```python
from build123d import *

# Parameters (mm, degrees)
F1_DEPTH = 9


with BuildPart() as f1:
    # F0 (on Front) → F1 (new body)
    with BuildSketch(Plane.XZ):
        with BuildLine():
            ThreePointArc((-19.7199515168, 22.7688088414), (-16.6360107994, 24.4598997459), (-13.1759548296, 25.0911615632))
            Line((-13.1759548296, 25.0911615632), (-12.553585429, 26.9574491451))
            Line((-12.553585429, 26.9574491451), (-10.2510419619, 28.9986901835))
            ThreePointArc((-10.2510419619, 28.9986901835), (-10.1077855778, 34.1050974839), (-7.8535185141, 38.6892220367))
            ThreePointArc((-7.8535185141, 38.6892220367), (-18.8089000647, 34.4723344318), (-19.7199515168, 22.7688088414))
        make_face()
        with BuildLine():
            Line((-14.8518085926, 20.0658099574), (-13.1759548296, 25.0911615632))
            ThreePointArc((-13.1759548296, 25.0911615632), (-16.6360107994, 24.4598997459), (-19.7199515168, 22.7688088414))
            ThreePointArc((-19.7199515168, 22.7688088414), (-17.4770465825, 19.8404198684), (-14.3921665295, 17.8181440266))
            Line((-14.3921665295, 17.8181440266), (-14.8518085926, 20.0658099574))
        make_face()
        with BuildLine():
            Line((-13.3963086419, 12.9483637654), (-14.3921665295, 17.8181440266))
            ThreePointArc((-14.3921665295, 17.8181440266), (-17.4770465825, 19.8404198684), (-19.7199515168, 22.7688088414))
            ThreePointArc((-19.7199515168, 22.7688088414), (-22.6703383342, 8.9306933135), (-9.5498657155, 3.6343339981))
            ThreePointArc((-9.5498657155, 3.6343339981), (-12.2712093358, 7.7530477474), (-13.1041599616, 12.6188166798))
            Line((-13.1041599616, 12.6188166798), (-13.3963086419, 12.9483637654))
        make_face()
        with BuildLine():
            Line((-3.2264382129, 0.3550507135), (-3.2264382129, 5.7278911556))
            Line((-3.2264382129, 5.7278911556), (-5.1312660195, 6.3631129466))
            ThreePointArc((-5.1312660195, 6.3631129466), (-7.1772197402, 4.7342237961), (-9.5498657155, 3.6343339981))
            ThreePointArc((-9.5498657155, 3.6343339981), (-6.6370818502, 1.5146819538), (-3.2264382129, 0.3550507135))
        make_face()
        with BuildLine():
            Line((-1.6854464257, 5.2140013649), (-3.2264382129, 5.7278911556))
            Line((-3.2264382129, 5.7278911556), (-3.2264382129, 0.3550507135))
            ThreePointArc((-3.2264382129, 0.3550507135), (0.2553267791, 0.2456421269), (3.6218142124, 1.140862803))
            Line((3.6218142124, 1.140862803), (3.5146783317, 6.277413876))
            Line((3.5146783317, 6.277413876), (-0.6090724081, 5.4341171602))
            Line((-0.6090724081, 5.4341171602), (-1.6854464257, 5.2140013649))
        make_face()
        with BuildLine():
            ThreePointArc((-9.5498657155, 3.6343339981), (-7.1772197402, 4.7342237961), (-5.1312660195, 6.3631129466))
            Line((-5.1312660195, 6.3631129466), (-8.5770856134, 7.5122245284))
            Line((-8.5770856134, 7.5122245284), (-13.1041599616, 12.6188166798))
            ThreePointArc((-13.1041599616, 12.6188166798), (-12.2712093358, 7.7530477474), (-9.5498657155, 3.6343339981))
        make_face()
        with BuildLine():
            ThreePointArc((3.6218142124, 1.140862803), (0.2553267791, 0.2456421269), (-3.2264382129, 0.3550507135))
            Line((-3.2264382129, 0.3550507135), (-3.2264382129, -30.5104665458))
            Line((-3.2264382129, -30.5104665458), (0, -30.5104665458))
            Line((0, -30.5104665458), (4.2804706275, -30.4379349907))
            Line((4.2804706275, -30.4379349907), (3.6218142124, 1.140862803))
        make_face()
        with BuildLine():
            ThreePointArc((-7.8535185141, 38.6892220367), (-10.1077855778, 34.1050974839), (-10.2510419619, 28.9986901835))
            Line((-10.2510419619, 28.9986901835), (-7.117446192, 31.7766721736))
            Line((-7.117446192, 31.7766721736), (-0.3315885654, 33.1643630917))
            ThreePointArc((-0.3315885654, 33.1643630917), (-3.477568869, 36.7640757707), (-7.8535185141, 38.6892220367))
        make_face()
        with BuildLine():
            ThreePointArc((12.5130116372, 36.0825908768), (3.0643977065, 43.1259953977), (-7.8535185141, 38.6892220367))
            ThreePointArc((-7.8535185141, 38.6892220367), (-3.477568869, 36.7640757707), (-0.3315885654, 33.1643630917))
            Line((-0.3315885654, 33.1643630917), (0, 33.2321721243))
            Line((0, 33.2321721243), (2.4402343405, 32.4184030146))
            ThreePointArc((2.4402343405, 32.4184030146), (7.0001300905, 35.5603661525), (12.5130116372, 36.0825908768))
        make_face()
        with BuildLine():
            Line((3.5146783317, 6.277413876), (3.6218142124, 1.140862803))
            ThreePointArc((3.6218142124, 1.140862803), (4.1675414436, 1.3915355093), (4.70004417, 1.6691969268))
            Line((4.70004417, 1.6691969268), (4.70004417, 5.4740770661))
            ThreePointArc((4.70004417, 5.4740770661), (4.1944674507, 5.8815460805), (3.7138142861, 6.3181366808))
            Line((3.7138142861, 6.3181366808), (3.5146783317, 6.277413876))
        make_face()
        with BuildLine():
            ThreePointArc((20.5664608958, 20.2387270332), (20.5664608958, 30.2074464559), (12.5130116372, 36.0825908768))
            ThreePointArc((12.5130116372, 36.0825908768), (13.5239296541, 30.5833992601), (11.9332966326, 25.2230867446))
            ThreePointArc((11.9332966326, 25.2230867446), (16.8469164385, 23.7650064749), (20.5664608958, 20.2387270332))
        make_face()
        with BuildLine():
            ThreePointArc((11.9332966326, 25.2230867446), (13.5239296541, 30.5833992601), (12.5130116372, 36.0825908768))
            ThreePointArc((12.5130116372, 36.0825908768), (7.0001300905, 35.5603661525), (2.4402343405, 32.4184030146))
            Line((2.4402343405, 32.4184030146), (6.8916391877, 30.9339489607))
            Line((6.8916391877, 30.9339489607), (11.7108622162, 25.4978097237))
            Line((11.7108622162, 25.4978097237), (11.7654730156, 25.2307609848))
            ThreePointArc((11.7654730156, 25.2307609848), (11.849399475, 25.2272442579), (11.9332966326, 25.2230867446))
        make_face()
        with BuildLine():
            Line((4.70004417, 5.4740770661), (4.70004417, 1.6691969268))
            ThreePointArc((4.70004417, 1.6691969268), (6.2285853657, 2.6749839802), (7.5864404314, 3.9014730362))
            ThreePointArc((7.5864404314, 3.9014730362), (6.0841704451, 4.579353109), (4.70004417, 5.4740770661))
        make_face()
        with BuildLine():
            Line((5.4319997663, 6.6695013155), (4.70004417, 6.5198182262))
            Line((4.70004417, 6.5198182262), (4.70004417, 5.4740770661))
            ThreePointArc((4.70004417, 5.4740770661), (6.0841704451, 4.579353109), (7.5864404314, 3.9014730362))
            ThreePointArc((7.5864404314, 3.9014730362), (9.9012477971, 7.4035929552), (10.8681390033, 11.488724344))
            Line((10.8681390033, 11.488724344), (5.4319997663, 6.6695013155))
        make_face()
        with BuildLine():
            ThreePointArc((20.5664608958, 20.2387270332), (16.8469164385, 23.7650064749), (11.9332966326, 25.2230867446))
            ThreePointArc((11.9332966326, 25.2230867446), (11.8720696964, 25.1182665807), (11.8097855463, 25.0140711437))
            Line((11.8097855463, 25.0140711437), (13.1663621669, 18.3803635317))
            Line((13.1663621669, 18.3803635317), (11.7962916439, 14.2719584578))
            ThreePointArc((11.7962916439, 14.2719584578), (16.9481115684, 16.1283678588), (20.5664608958, 20.2387270332))
        make_face()
        with BuildLine():
            ThreePointArc((7.5864404314, 3.9014730362), (19.9595132668, 7.3959808102), (20.5664608958, 20.2387270332))
            ThreePointArc((20.5664608958, 20.2387270332), (16.9481115684, 16.1283678588), (11.7962916439, 14.2719584578))
            Line((11.7962916439, 14.2719584578), (10.8681390033, 11.488724344))
            ThreePointArc((10.8681390033, 11.488724344), (9.9012477971, 7.4035929552), (7.5864404314, 3.9014730362))
        make_face()
    extrude(amount=F1_DEPTH)


solid = f1.part
```
Build history of the part. All positions in model axes, mm. A direction names the side the tool comes from. Round coordinates to 2 decimals unless told otherwise and drop trailing zeros. Write each loop counter-clockwise with the first axis right and the second up, starting at its lowest first coordinate (ties: lowest second). Pieces come first, ordered by that corner, then holes. Notation, with made-up numbers: (-25.75, -21) - (-21.75, -21) arc R25 ccw to (-21.75, -2) - close; hole circle Ø7 at (50, 82.5). An arc over 180 degrees is marked (long way). Write each question's results on one line, items separated by ' | '. Start each with the question number.
Item 1: Saw through at D-D (x = 18.5). Write the cut outline in (y, z).
Item 2: Drop flat-ended pins along their axis: P1, Ø3, axis at y = -6.5, z = 20, coming from the -X side; P2, Ø1.2, axis at y = -6, z = 6, coming from the -X side; P3, Ø6, axis at x = -8.5, z = -22, coming from the -Y side; P4, Ø1, axis at x = -10, y = -4, coming from the +Z side. Give the stop position or say it passes through.
Item 3: Wall check: L1, parallel to Z at x = 0.5, y = -0.75; L2, parallel to Z at x = 9.5, y = -3.25; L3, parallel to X at y = -2.5, z = 30. Give the ranges that are in metal, low to high. Write a range as [from, to].
Item 4: Saw through at A-A (x = 10). Write the cut outline in (y, z), and give its area (3 significant figures).
Item 5: Mould opens along Z. For faces 1 (the face through (12.48, -4.44, 21.74)), 2 (the face through (-2, -4, -30.51)), 3 (the face through (5.9, -9, 6.5)), 4 (the face through (3.235, -4.437, 43.103)) say: pulls with the +Z half, pulls with the -Z half, needs draft (parallel to the pull), parting line crosses it, or undercut.
Item 6: Saw through at C-C (z = -14). Write the cut outline in (x, y), and give its area (3 significant figures).
Item 7: Saw through at B-B (z = 24). Write the cut outline in (x, y), and give its area (3 significant figures).
Item 8: Which spindle directions (+Z, -Z, +X, -X, +Y, -Y) get a long thin tool onto all of the face, cutting with end or side? Do faces 5 (the face through (-3.226, -4, -15)), 6 (the face through (8.188, -4.437, 9.113)), 7 (the face through (20.63, -4.44, 30.08)). Say none if no direction does.
Results are:
1) outline: (-9, 5.88) - (0, 5.88) - (0, 33.04) - (-9, 33.04) - close
2) P1: stops at x = -23.04 | P2: stops at x = -21.01 | P3: passes through | P4: stops at z = 38.9
3) L1: z = [-30.5, 5.66], [33.07, 43.18] | L2: z = [3.39, 10.28], [27.99, 40.2] | L3: x = [-20.79, -9.12], [7.72, 20.67]
4) outline: (-9, 3.32) - (0, 3.32) - (0, 10.72) - (-9, 10.72) - close; (-9, 27.43) - (0, 27.43) - (0, 39.73) - (-9, 39.73) - close | area: 177 mm²
5) face 1: undercut | face 2: pulls with the -Z half | face 3: needs draft | face 4: pulls with the +Z half
6) outline: (-3.23, -9) - (3.94, -9) - (3.94, 0) - (-3.23, 0) - close | area: 64.5 mm²
7) outline: (-20.28, -9) - (-13.54, -9) - (-13.54, 0) - (-20.28, 0) - close; (12.02, -9) - (21.69, -9) - (21.69, 0) - (12.02, 0) - close | area: 148 mm²
8) face 5: -Z, -X, +Y, -Y | face 6: +Y, -Y | face 7: +X, +Y, -Y
